Here's how the part is built. I have some questions about the finished solid (model axes, mm). Round coordinates to 2 decimals unless told otherwise and drop trailing zeros. Loops run counter-clockwise (first coordinate to the right, second up) from the corner with the lowest first, then second, coordinate; pieces in that order, holes last. Notation, with made-up numbers: M 43.5,42 L 66.5,42 A11 ccw 66.5,57 Z; hole C 29,49 d1. An arc over 180 degrees is marked long. Write each question's results on one line, items separated by ' | '. Start each with the question number.
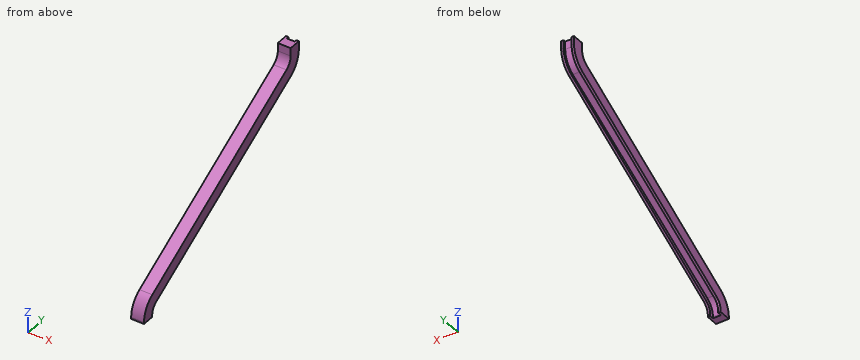
```python
from build123d import *

# Parameters (mm, degrees)
BOSS_EXTRUDE1_DEPTH = 16
CUT_EXTRUDE1_START  = -13
CUT_EXTRUDE1_DEPTH  = 10


with BuildPart() as part:
    # Sketch1 → Boss-Extrude1 (new body)
    with BuildSketch(Plane(origin=(0, 0, 0), x_dir=(0, 0, -1), z_dir=(1, 0, 0))):
        with BuildLine():
            Line((0, 0), (10, 0))
            ThreePointArc((10, 0), (17.565310247, -2.047545373), (23.065245029, -7.631189218))
            Line((23.065245029, -7.631189218), (161.869509942, -253.737621564))
            ThreePointArc((161.869509942, -253.737621564), (172.869379506, -264.904909254), (188, -269))
            Line((188, -269), (190, -269))
            Line((190, -269), (190, -254))
            Line((190, -254), (188, -254))
            ThreePointArc((188, -254), (180.434689753, -251.952454627), (174.934754971, -246.368810782))
            Line((174.934754971, -246.368810782), (36.130490058, -0.262378436))
            ThreePointArc((36.130490058, -0.262378436), (25.130620494, 10.904909254), (10, 15))
            Line((10, 15), (0, 15))
            Line((0, 15), (0, 0))
        make_face()
    extrude(amount=BOSS_EXTRUDE1_DEPTH)

    # Sketch3 → Cut-Extrude1 (cut)
    with BuildSketch(Plane(origin=(16, 0, 0), x_dir=(0, 0, -1), z_dir=(1, 0, 0)).offset(CUT_EXTRUDE1_START)):
        with BuildLine():
            Line((10, 15), (0, 15))
            Line((0, 15), (0, 12))
            Line((0, 12), (10, 12))
            ThreePointArc((10, 12), (23.700034196, 8.26604958), (33.610790729, -1.903032367))
            Line((33.610790729, -1.903032367), (170.510525386, -248.701457506))
            ThreePointArc((170.510525386, -248.701457506), (177.851826522, -256.2341108), (188, -259))
            Line((188, -259), (190, -259))
            Line((190, -259), (190, -254))
            Line((190, -254), (188, -254))
            ThreePointArc((188, -254), (180.434689753, -251.952454627), (174.934754971, -246.368810782))
            Line((174.934754971, -246.368810782), (36.130490058, -0.262378436))
            ThreePointArc((36.130490058, -0.262378436), (25.130620494, 10.904909254), (10, 15))
        make_face()
    extrude(amount=CUT_EXTRUDE1_DEPTH, mode=Mode.SUBTRACT)


solid = part.part
```
Item 1: I need wall thicknesses on L1, parallel to Y at x = 9, z = -10; L2, parallel to Z at x = 7.5, y = -125.5; L3, parallel to Y at x = 12.75, z = -165.5. Which ranges of each line are inside material? Lowest first, please.
Item 2: I'm going to push flat-ended pins straight in: pin 1 (4 mm diameter, centred on x = 10.5, y = -156.5, fed in from -Z); pin 2 (8 mm diameter, centred on x = 12.5, z = -105, fed in from -Y); pin 3 (3 mm diameter, centred on x = 13, z = -97.5, fed in from +Y). Where does each tip first touch, or does it pass through?
Item 3: If we section it at B-B on z = -115.5: Please give me the cut outline in (x, y), and give its area (3 significant figures).
Item 4: If we section it at C-C on y = -101.5: Please give me the cut outline in (x, z), and give its area (3 significant figures).
Item 5: If we section it at A-A on x = 5.5: Please give me the cut outline in (y, z).
Numbers:
1) L1: 0 to 12 | L2: -102.17 to -89.54 | L3: -258.84 to -239.67
2) pin 1: z = -120.48 | pin 2: y = -160 | pin 3: y = -106.41
3) outline: M 0,-171.52 L 16,-171.52 L 16,-140.99 L 13,-140.99 L 13,-149.53 L 3,-149.53 L 3,-140.99 L 0,-140.99 Z | area: 403 mm²
4) outline: M 0,-93.23 L 3,-93.23 L 3,-88.86 L 13,-88.86 L 13,-93.23 L 16,-93.23 L 16,-76.01 L 0,-76.01 Z | area: 232 mm²
5) outline: M -269,-190 L -259,-190 L -259,-188 A20 cw -248.7,-170.51 L -1.9,-33.61 A27 ccw 12,-10 L 12,0 L 0,0 L 0,-10 A15 cw -7.63,-23.07 L -253.74,-161.87 A30 ccw -269,-188 Z
